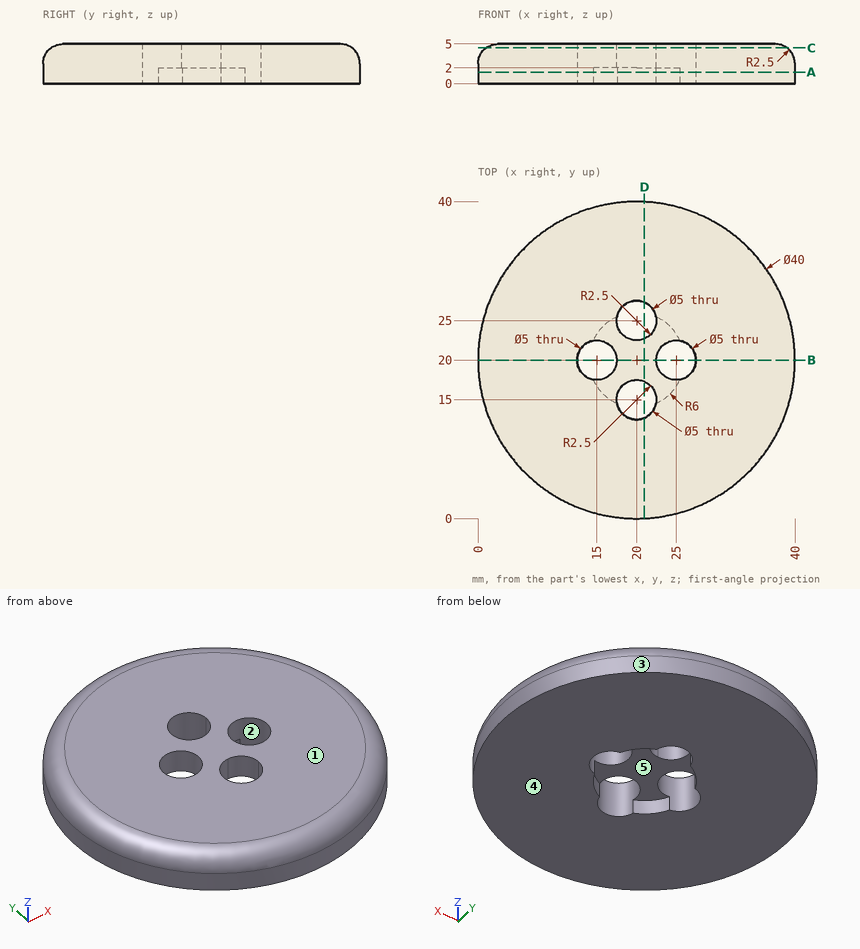
Input: dimensioned drawing with shaded views. Units: mm. Origin: part minimum x, y, z. A direction names the side the tool comes from. Coordinates: 2 decimals unless noted, no trailing zeros. Loops run counter-clockwise (first coordinate to the right, second up) from the corner with the lowest first, then second, coordinate; pieces in that order, holes last.
Q1. Contact query for flat-ended pins moving along their axis: pin 1 (4 mm diameter, centred on x = 20, y = 25, fed in from +Z); pin 2 (5.5 mm diameter, centred on x = 20, y = 21, fed in from -Z); pin 3 (2 mm diameter, centred on x = 20.5, z = 1, fed in from +Y). Output: stop coordinate, or through.
Results are:
pin 1: passes through
pin 2: stops at z = 2
pin 3: stops at y = 40
Q2. Section A-A, the plane z = 1.45. Return the cut outline in (x, y) (3 decimals).
Results are:
outline: circle Ø40 at (20, 20); hole (14.525, 17.546) arc R6 ccw to (17.546, 14.525) arc R2.5 ccw to (22.454, 14.525) arc R6 ccw to (25.475, 17.546) arc R2.5 ccw to (25.475, 22.454) arc R6 ccw to (22.454, 25.475) arc R2.5 ccw to (17.546, 25.475) arc R6 ccw to (14.525, 22.454) arc R2.5 ccw to start
Q3. Section B-B, the plane y = 20. Return the cut outline in (x, z).
Results are:
outline: (0, 0) - (12.5, 0) - (12.5, 5) - (2.5, 5) arc R2.5 ccw to (0, 2.5) - close; (17.5, 2) - (22.5, 2) - (22.5, 5) - (17.5, 5) - close; (27.5, 0) - (40, 0) - (40, 2.5) arc R2.5 ccw to (37.5, 5) - (27.5, 5) - close
Q4. Section C-C, the plane z = 4.5. Return the cut outline in (x, y).
Results are:
outline: circle Ø38 at (20, 20); hole circle Ø5 at (15, 20); hole circle Ø5 at (20, 15); hole circle Ø5 at (20, 25); hole circle Ø5 at (25, 20)
Q5. Set-up query: the marked faces 4 and 5. Return all of +Z, -Z, +X, -X, +Y, -Y with unobstructed straight access to the full face (end or side cutting, diameter ignored); none if empty.
Results are:
face 4: -Z, +X, -X, +Y, -Y
face 5: -Z
Q6. Line query: line 1 along Y through (x, z) = (20, 2.6); line 2 along Y through (x, z) = (20, 1.7); line 3 along Y through (x, z) = (21.5, 3.5). Output: solid intervals per line, ascending.
Results are:
line 1: y = 0 to 12.5, 17.5 to 22.5, 27.5 to 40
line 2: y = 0 to 12.5, 27.5 to 40
line 3: y = 0.27 to 13, 17 to 23, 27 to 39.73
Q7. Section D-D, the plane x = 21. Give the number of separate pieces and of enclosed holes in the cut face, and give its area (3 significant figures).
Results are:
separate pieces: 3
enclosed holes: 0
area: 140 mm2
Q8. Mould query, pull axis Y, two halves, no side actions, for the marked faces 1, 2 and 3. Classes: +Y half, -Y half, draft (parallel to the pull), parting line (faces both ways), or undercut.
Results are:
face 1: draft
face 2: undercut
face 3: parting line
